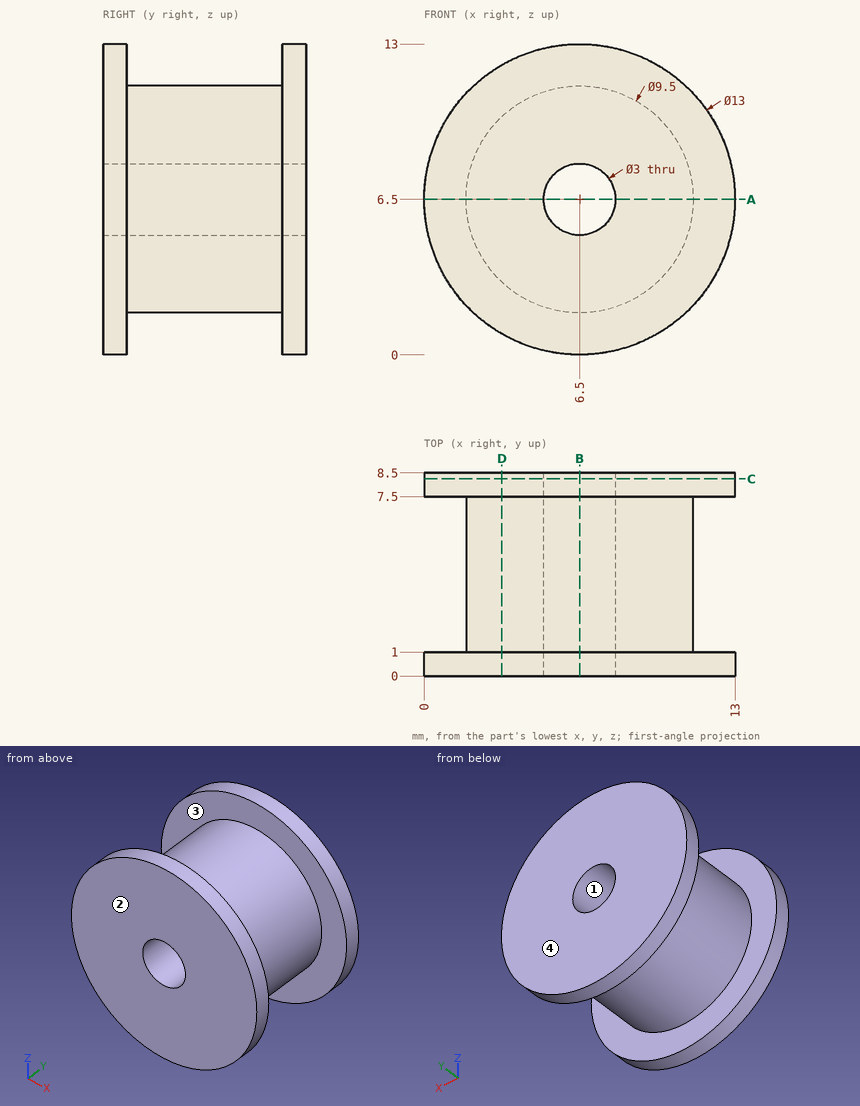
The figure shows three views and two pictorial views of one solid part (mm, origin at its lowest corner). Answer the questions. Round coordinates to 2 decimals unless told otherwise and drop trailing zeros. Order: outer loops, then holes, each group sorted by start corner. A loop starts at its lowest first (then second) coordinate and runs counter-clockwise, first axis right, second up. Notation, with made-up numbers: M 54.25,0.5 L 80.25,0.5 A27 ccw 80.25,16.5 Z; hole C 52,17 d9. An arc over 180 degrees is marked long. Put each result on its own line as item: value. Start each with the question number.
Q1. Section C-C, the plane y = 8.25 is taken. Write down the section's boundary in (x, z), and give its area (3 significant figures).
Q2. Section A-A, the plane z = 6.5 is taken. Write down the section's boundary in (x, y), and give its area (4 significant figures).
Q3. Flat-ended cylindrical pins translate along their axes: pin 1 (1 mm diameter, centred on y = 6.5, z = 6, fed in from +X); pin 2 (4 mm diameter, centred on x = 2, y = 1.5, fed in from +Z); pin 3 (5 mm diameter, centred on x = 5, y = 4.5, fed in from -Z). Find the tip coordinate at first contact, or state that the pin passes through.
Q4. For a pull along Y with two mould halves and no side action, classify the marked faces 1, 2, 3 and 4 as pulls with the +Y half, pulls with the -Y half, needs draft (parallel to the pull), parting line crosses it, or undercut.
Q5. Straight lines are drawn through the part: L1, parallel to Z at x = 6.5, y = 6.25; L2, parallel to Y at x = 1.5, z = 6. For each, find the intervals that lie inside material, in ascending order. Write a range as [from, to].
Q6. Section B-B, the plane x = 6.5 is taken. Write down the section's boundary in (y, z).
Q7. Section D-D, the plane x = 3.25 is taken. Write down the section's boundary in (y, z), and give its area (4 significant figures).
Findings below:
1. outline: C 6.5,6.5 d13; hole C 6.5,6.5 d3
1. area: 126 mm^2
2. outline: M 0,0 L 5,0 L 5,8.5 L 0,8.5 L 0,7.5 L 1.75,7.5 L 1.75,1 L 0,1 Z; M 8,0 L 13,0 L 13,1 L 11.25,1 L 11.25,7.5 L 13,7.5 L 13,8.5 L 8,8.5 Z
2. area: 62.25 mm^2
3. pin 1: stops at x = 11.25
3. pin 2: stops at z = 12.47
3. pin 3: stops at z = 1.75
4. face 1: needs draft
4. face 2: pulls with the -Y half
4. face 3: undercut
4. face 4: pulls with the +Y half
5. L1: z = [1.75, 5], [8, 11.25]
5. L2: y = [0, 1], [7.5, 8.5]
6. outline: M 0,0 L 1,0 L 1,1.75 L 7.5,1.75 L 7.5,0 L 8.5,0 L 8.5,5 L 0,5 Z; M 0,8 L 8.5,8 L 8.5,13 L 7.5,13 L 7.5,11.25 L 1,11.25 L 1,13 L 0,13 Z
7. outline: M 0,0.87 L 1,0.87 L 1,3.04 L 7.5,3.04 L 7.5,0.87 L 8.5,0.87 L 8.5,12.13 L 7.5,12.13 L 7.5,9.96 L 1,9.96 L 1,12.13 L 0,12.13 Z
7. area: 67.55 mm^2
